Build history of the part. All positions in model axes, mm. Coordinates: 2 decimals unless noted, no trailing zeros. Order: outer loops, then holes, each group sorted by start corner. A loop starts at its lowest first (then second) coordinate and runs counter-clockwise, first axis right, second up. Notation, with made-up numbers: (23.5, 14) -> (57.5, 14) arc R14 cw to (57.5, 19) -> close; hole circle Ø2 at (-35.75, 31). An arc over 180 degrees is marked (long way). Write each question's results on one line, items separated by ' | '.
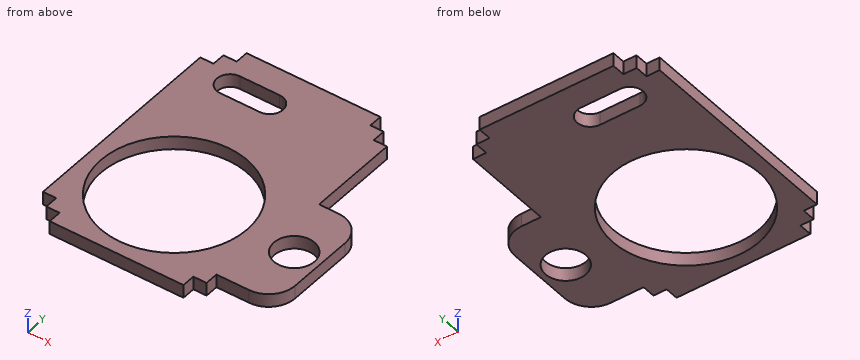
from build123d import *

# Parameters (mm, degrees)
SKETCH1_R           = 35.1155
SKETCH1_R_2         = 9.7234375
BOSS_EXTRUDE1_DEPTH = 6.35
CUT_EXTRUDE1_DEPTH  = 114.602654559


with BuildPart() as part:
    # Sketch1 → Boss-Extrude1 (new body)
    with BuildSketch(Plane.XY):
        with BuildLine():
            Line((75.062413888, -16.133650292), (75.062413888, 15.997349708))
            ThreePointArc((75.062413888, 15.997349708), (71.342670009, 24.977605829), (62.362413888, 28.697349708))
            Line((62.362413888, 28.697349708), (53.104113888, 28.697349708))
            Line((53.104113888, 28.697349708), (53.104113888, 72.334549708))
            Line((53.104113888, 72.334549708), (46.754113888, 72.334549708))
            Line((46.754113888, 72.334549708), (46.754113888, 78.684549708))
            Line((46.754113888, 78.684549708), (40.404113888, 78.684549708))
            Line((40.404113888, 78.684549708), (40.404113888, 85.034549708))
            Line((40.404113888, 85.034549708), (-23.883286112, 85.034549708))
            Line((-23.883286112, 85.034549708), (-23.883286112, 78.684549708))
            Line((-23.883286112, 78.684549708), (-30.233286112, 78.684549708))
            Line((-30.233286112, 78.684549708), (-30.233286112, 72.334549708))
            Line((-30.233286112, 72.334549708), (-36.583286112, 72.334549708))
            Line((-36.583286112, 72.334549708), (-36.583286112, -28.833650292))
            Line((-36.583286112, -28.833650292), (-30.233286112, -28.833650292))
            Line((-30.233286112, -28.833650292), (-30.233286112, -35.183650292))
            Line((-30.233286112, -35.183650292), (-23.883286112, -35.183650292))
            Line((-23.883286112, -35.183650292), (-23.883286112, -41.533650292))
            Line((-23.883286112, -41.533650292), (40.404113888, -41.533650292))
            Line((40.404113888, -41.533650292), (40.404113888, -35.183650292))
            Line((40.404113888, -35.183650292), (46.754113888, -35.183650292))
            Line((46.754113888, -35.183650292), (46.754113888, -28.833650292))
            Line((46.754113888, -28.833650292), (62.362413888, -28.833650292))
            ThreePointArc((62.362413888, -28.833650292), (71.342670009, -25.113906413), (75.062413888, -16.133650292))
        make_face()
        with Locations((4.882213888, -0.068150292)):
            Circle(SKETCH1_R, mode=Mode.SUBTRACT)
        with Locations((62.629113888, -0.068150292)):
            Circle(SKETCH1_R_2, mode=Mode.SUBTRACT)
    extrude(amount=-BOSS_EXTRUDE1_DEPTH)

    # Sketch2 → Cut-Extrude1 (cut, through all)
    with BuildSketch(Plane.XY):
        with BuildLine():
            Line((-17.533286112, 59.634549708), (1.516713888, 59.634549708))
            ThreePointArc((1.516713888, 59.634549708), (7.866713888, 65.984549708), (1.516713888, 72.334549708))
            Line((1.516713888, 72.334549708), (-17.533286112, 72.334549708))
            ThreePointArc((-17.533286112, 72.334549708), (-23.883286112, 65.984549708), (-17.533286112, 59.634549708))
        make_face()
    extrude(amount=-CUT_EXTRUDE1_DEPTH, mode=Mode.SUBTRACT)


solid = part.part
Item 1: Pin check, flat tips, straight feed: pin 1 (3 mm diameter, centred on y = 74, z = -3, fed in from -X); pin 2 (3 mm diameter, centred on y = 82, z = -2.5, fed in from +X); pin 3 (3 mm diameter, centred on x = 55.5, z = -2.5, fed in from +Y). Stop position of each tip, or through.
Answer:
pin 1: stops at x = -30.23 | pin 2: stops at x = 40.4 | pin 3: stops at y = 28.7
Item 2: Slice it at C-C, the plane y = -32.5. List the corners of the cut face in (x, z).
Answer:
outline: (-30.23, -6.35) -> (-8.58, -6.35) -> (-8.58, 0) -> (-30.23, 0) -> close; (18.35, -6.35) -> (46.75, -6.35) -> (46.75, 0) -> (18.35, 0) -> close
Item 3: Slice it at B-B, the plane z = -3. State how many separate pieces and enclosed holes the cut face has, and give its area (3 significant figures).
Answer:
separate pieces: 1 | enclosed holes: 3 | area: 7,520 mm^2
Item 4: Slice it at D-D, the plane x = 23. List the corners of the cut face in (y, z), and give its area (3 significant figures).
Answer:
outline: (-41.53, -6.35) -> (-30.15, -6.35) -> (-30.15, 0) -> (-41.53, 0) -> close; (30.01, -6.35) -> (85.03, -6.35) -> (85.03, 0) -> (30.01, 0) -> close | area: 422 mm^2
Item 5: Drill centre lines: line 1 (Y direction, x = -19.5, z = -1); line 2 (X direction, y = 2, z = -4.5); line 3 (Y direction, x = -18.5, z = -5). Where is each one in solid material? Low to high. Write a range as from..to.
Answer:
line 1: y = -41.53..-25.34, 25.2..59.95, 72.02..85.03 | line 2: x = -36.58..-30.17, 39.94..53.13, 72.13..75.06 | line 3: y = -41.53..-26.27, 26.13..59.71, 72.26..85.03
Item 6: Slice it at A-A, the plane x = 5.5. List the corners of the cut face in (y, z), and give its area (3 significant figures).
Answer:
outline: (-41.53, -6.35) -> (-35.18, -6.35) -> (-35.18, 0) -> (-41.53, 0) -> close; (35.04, -6.35) -> (61.04, -6.35) -> (61.04, 0) -> (35.04, 0) -> close; (70.93, -6.35) -> (85.03, -6.35) -> (85.03, 0) -> (70.93, 0) -> close | area: 295 mm^2
